```python
from build123d import *

# Parameters (mm, degrees)
SKETCH1_R           = 31.75
SKETCH1_R_2         = 21.59
BOSS_EXTRUDE1_DEPTH = 5.08
SKETCH2_R           = 31.75
BOSS_EXTRUDE2_DEPTH = 2.54
SKETCH3_R           = 1.7272
CUT_EXTRUDE1_DEPTH  = 7.62
SKETCH4_R           = 6.35
CUT_EXTRUDE2_DEPTH  = 2.54


with BuildPart() as part:
    # Sketch1 → Boss-Extrude1 (new body)
    with BuildSketch(Plane.XY):
        Circle(SKETCH1_R)
        Circle(SKETCH1_R_2, mode=Mode.SUBTRACT)
    extrude(amount=BOSS_EXTRUDE1_DEPTH)

    # Sketch2 → Boss-Extrude2 (add)
    with BuildSketch(Plane.XY.offset(5.08)):
        Circle(SKETCH2_R)
    extrude(amount=BOSS_EXTRUDE2_DEPTH)

    # Sketch3 → Cut-Extrude1 (cut)
    with BuildSketch(Plane(origin=(0, 0, 0), x_dir=(-1, 0, 0), z_dir=(0, 0, -1))):
        with Locations((0, 28.575)):
            Circle(SKETCH3_R)
        with Locations((28.575, 0)):
            Circle(SKETCH3_R)
        with Locations((0, -28.575)):
            Circle(SKETCH3_R)
        with Locations((-28.575, 0)):
            Circle(SKETCH3_R)
    extrude(amount=-CUT_EXTRUDE1_DEPTH, mode=Mode.SUBTRACT)

    # Sketch4 → Cut-Extrude2 (cut)
    with BuildSketch(Plane.XY.offset(7.62)):
        Circle(SKETCH4_R)
    extrude(amount=-CUT_EXTRUDE2_DEPTH, mode=Mode.SUBTRACT)


solid = part.part
```
The model under review builds one solid part; all positions refer to its coordinate system, in mm. A direction names the side the tool comes from. Round coordinates to 2 decimals unless told otherwise and drop trailing zeros. Write each loop counter-clockwise with the first axis right and the second up, starting at its lowest first coordinate (ties: lowest second). Pieces come first, ordered by that corner, then holes.
(1) We need section D-D on y = -10.5. Give the boundary of the cut face in (x, z), and give its area (3 significant figures).
(2) Machinability: for faces 1 (the cylindrical face through (-15.913, 14.592, 2.504)), 2 (the cylindrical face through (0.22, -26.86, 3.76)), which of the approach directions +Z, -Z, +X, -X, +Y, -Y give a long, thin tool a straight path to every point of the face, cutting with its end or side? Answer none if there is none.
(3) Mouldability with a two-part tool opening along Y and no side actions: class faces 3 (the cylindrical face through (-6.883, -30.995, 3.757)), 4 (the flat face through (7, 0, 7.62)), 5 (the cylindrical face through (0.22, 30.29, 3.76)) as +Y half, -Y half, draft (parallel to the pull), parting line (faces both ways), or undercut.
(4) We need section C-C on z = 4. Give the boundary of the cut face in (x, y) (3 decimals).
(5) We need section A-A on x = 0. Give the boundary of the cut face in (y, z), and give its area (3 significant figures).
(6) Wall thickness on L1, parallel to Y at x = 0, z = 3.75; L2, parallel to Y at x = 0, z = 5.5; L3, parallel to Z at x = 4.5, y = 18.5: over which ranges is each line inside the solid? List them lowest first.
(7) Insertion check: pin 1 (3 mm diameter, centred on x = 0, y = 28.575, fed in from -Z); pin 2 (4 mm diameter, centred on x = -28.575, y = 0, fed in from -Z); pin 3 (21.5 mm diameter, centred on x = -6, y = -2.5, fed in from -Z); pin 4 (3 mm diameter, centred on y = -24.5, z = 1.5, fed in from +X). Each pin has a flat end and moves straight along its axis. Give the tip position at first contact, or say it passes through.
Findings below:
1. outline: (-29.96, 0) - (-18.86, 0) - (-18.86, 5.08) - (18.86, 5.08) - (18.86, 0) - (29.96, 0) - (29.96, 7.62) - (-29.96, 7.62) - close
1. area: 265 mm2
2. face 1: -Z
2. face 2: +Z, -Z
3. face 3: parting line
3. face 4: draft
3. face 5: undercut
4. outline: circle Ø63.5 at (0, 0); hole circle Ø3.454 at (-28.575, 0); hole circle Ø43.18 at (0, 0); hole circle Ø3.454 at (0, -28.575); hole circle Ø3.454 at (0, 28.575); hole circle Ø3.454 at (28.575, 0)
5. outline: (-31.75, 0) - (-30.3, 0) - (-30.3, 7.62) - (-31.75, 7.62) - close; (-26.85, 0) - (-21.59, 0) - (-21.59, 5.08) - (-6.35, 5.08) - (-6.35, 7.62) - (-26.85, 7.62) - close; (6.35, 5.08) - (21.59, 5.08) - (21.59, 0) - (26.85, 0) - (26.85, 7.62) - (6.35, 7.62) - close; (30.3, 0) - (31.75, 0) - (31.75, 7.62) - (30.3, 7.62) - close
5. area: 180 mm2
6. L1: y = -31.75 to -30.3, -26.85 to -21.59, 21.59 to 26.85, 30.3 to 31.75
6. L2: y = -31.75 to -30.3, -26.85 to -6.35, 6.35 to 26.85, 30.3 to 31.75
6. L3: z = 5.08 to 7.62
7. pin 1: passes through
7. pin 2: stops at z = 0
7. pin 3: stops at z = 5.08
7. pin 4: stops at x = 21.89
